from build123d import *

# Parameters (mm, degrees)
SKETCH1_R           = 10
BOSS_EXTRUDE1_DEPTH = 10.62
SKETCH3_R           = 3
CUT_EXTRUDE1_DEPTH  = 5
CUT_EXTRUDE1_DRAFT  = -2.25
DOME1_FACE_RADIUS   = 2.803549465
DOME1_HEIGHT        = 1


with BuildPart() as part:
    # Sketch1 → Boss-Extrude1 (new body)
    with BuildSketch(Plane(origin=(0, 0, 0), x_dir=(1, 0, 0), z_dir=(0, 1, 0))):
        with Locations(Location((0, 0, 0), (0, 0, 270))):
            Circle(SKETCH1_R)
    extrude(amount=BOSS_EXTRUDE1_DEPTH)

    # Sketch2 → Cut-Revolve1 (revolve, cut)
    with BuildSketch(Plane(origin=(0, 0, 0), x_dir=(0, 0, -1), z_dir=(1, 0, 0))):
        Polygon((11, 9.89), (10, 9.89), (10, 8.34), (3, 0), (11, 0), align=None)
        Polygon((11, 10.62), (8.925, 10.62), (8.925, 9.89), (10, 9.89), (11, 9.89), align=None)
    revolve(axis=Axis((0, 0, 0), (0, 1, 0)), mode=Mode.SUBTRACT)


with BuildPart() as cut_extrude1_tool:
    # Sketch3 → Cut-Extrude1 (with draft: the straight prism first)
    with BuildSketch(Plane.XZ):
        Circle(SKETCH3_R)
    extrude(amount=-CUT_EXTRUDE1_DEPTH)
    # Cut-Extrude1: the draft: its side faces are tilted about the plane it starts from
    cut_extrude1_sides = [cut_extrude1_tool.faces().sort_by_distance(p)[0] for p in [
        (-3, 2.5, 0),
    ]]
    draft(cut_extrude1_sides, Plane.XZ, CUT_EXTRUDE1_DRAFT)


with BuildPart() as part_1:
    add(part.part)

    # Cut-Extrude1: cut by cut_extrude1_tool
    add(cut_extrude1_tool.part, mode=Mode.SUBTRACT)

    # Dome1: a dome of height H over a round flat face of radius A is a cap of a sphere of radius (A * A + H * H) / (2 * H)
    dome1_r = (DOME1_FACE_RADIUS * DOME1_FACE_RADIUS + DOME1_HEIGHT * DOME1_HEIGHT) / (2 * DOME1_HEIGHT)
    dome1_base = Plane((0, 5, 0), z_dir=(0, -1, 0))
    with Locations(dome1_base.offset(DOME1_HEIGHT - dome1_r)):
        dome1_ball = Sphere(dome1_r, mode=Mode.PRIVATE)
    add(split(dome1_ball, bisect_by=dome1_base, keep=Keep.TOP, mode=Mode.PRIVATE))


solid = part_1.part
CAD build for the part. Positions are in the model's coordinates, mm. A direction names the side the tool comes from. Round coordinates to 2 decimals unless told otherwise and drop trailing zeros. Loops run counter-clockwise (first coordinate to the right, second up) from the corner with the lowest first, then second, coordinate; pieces in that order, holes last.
(1) Cut at C-C (y = 1). Give the cut face in (x, z), plus the area to 3 significant figures.
(2) Cut at A-A (x = 0). Give the cut face in (y, z) (3 decimals), plus the area to 3 significant figures.
(3) Wall check: line 1 along Z through (x, y) = (-0.75, 4); line 2 along X through (y, z) = (3.25, -1); line 3 along Z through (x, y) = (-2.25, 2). Give the ranges that are in metal, low to high.
(4) Cut at D-D (y = 6.25). Give the cut face in (x, z).
(5) Two-plate mould, pull along X, no slides. Class faces 3 (the conical face through (-0.629, 2.465, -2.834)), 4 (the flat face through (-7, 9.89, -6)), 5 (the cylindrical face through (-9.76, 9.1, -2.17)): +X half, -X half, draft (parallel to the pull), parting line (faces both ways), or undercut.
(6) Which spindle directions (+Z, -Z, +X, -X, +Y, -Y) get a long thin tool onto all of the face, cutting with end or side? Do faces 1 (the flat face through (0, 10.62, 0)), 2 (the cylindrical face through (-0.392, 10.25, 8.916)). Say none if no direction does.
(7) Drop flat-ended pins along their axis: pin 1 (2 mm diameter, centred on x = 0.5, y = 2, fed in from -Z); pin 2 (3 mm diameter, centred on x = 7.5, y = 5.5, fed in from -Z); pin 3 (3 mm diameter, centred on x = 5.5, z = 7, fed in from -Y). Give the stop position or say it passes through.
(8) Cut at B-B (z = 0). Give the cut face in (x, y) (3 decimals), plus the area to 3 significant figures.
Findings below:
1. outline: circle Ø7.68 at (0, 0); hole circle Ø5.92 at (0, 0)
1. area: 18.8 mm2
2. outline: (0, -3) - (8.34, -10) - (9.89, -10) - (9.89, -8.925) - (10.62, -8.925) - (10.62, 8.925) - (9.89, 8.925) - (9.89, 10) - (8.34, 10) - (0, 3) - (5, 2.804) arc R4.43 ccw to (5, -2.804) - close
2. area: 127 mm2
3. line 1: z = -6.31 to -2.74, 2.74 to 6.31
3. line 2: x = -5.64 to -2.69, 2.69 to 5.64
3. line 3: z = -4.1 to -1.86, 1.86 to 4.1
4. outline: circle Ø16.49 at (0, 0)
5. face 3: undercut
5. face 4: draft
5. face 5: parting line
6. face 1: +Z, -Z, +X, -X, +Y
6. face 2: +Y
7. pin 1: stops at z = -5.5
7. pin 2: stops at z = -5.56
7. pin 3: stops at y = 5.24
8. outline: (-10, 8.34) - (-3, 0) - (-2.804, 5) arc R4.43 ccw to (2.804, 5) - (3, 0) - (10, 8.34) - (10, 9.89) - (8.925, 9.89) - (8.925, 10.62) - (-8.925, 10.62) - (-8.925, 9.89) - (-10, 9.89) - close
8. area: 127 mm2
